from build123d import *

# Parameters (mm, degrees)
SKETCH1_W           = 25.27
SKETCH1_H           = 23.36
SKETCH1_R           = 1.5
SKETCH1_W_2         = 12.27
SKETCH1_H_2         = 10.36
SKETCH1_W_3         = 4
BOSS_EXTRUDE1_DEPTH = 3


with BuildPart() as part:
    # Sketch1 → Boss-Extrude1 (new body)
    # profile 1 of 2: a face of its own
    with BuildSketch(Plane.XY):
        Rectangle(SKETCH1_W, SKETCH1_H)
        with Locations((-9.635, 8.68)):
            Circle(SKETCH1_R, mode=Mode.SUBTRACT)
        with Locations((-9.635, -8.68)):
            Circle(SKETCH1_R, mode=Mode.SUBTRACT)
        with Locations((9.635, -8.68)):
            Circle(SKETCH1_R, mode=Mode.SUBTRACT)
        with Locations((9.635, 8.68)):
            Circle(SKETCH1_R, mode=Mode.SUBTRACT)
        with Locations((-0.085, -0.04)):
            Rectangle(SKETCH1_W_2, SKETCH1_H_2, mode=Mode.SUBTRACT)
    # profile 2 of 2: a face of its own
    with BuildSketch(Plane.XY):
        with Locations((-0.635, -0.04)):
            Rectangle(SKETCH1_W_3, SKETCH1_H_2)
    extrude(amount=BOSS_EXTRUDE1_DEPTH)


solid = part.part
The listing builds one solid part. Answer for the finished solid, in the listing's coordinates (mm). A direction names the side the tool comes from. Round coordinates to 2 decimals unless told otherwise and drop trailing zeros. Write each loop counter-clockwise with the first axis right and the second up, starting at its lowest first coordinate (ties: lowest second). Pieces come first, ordered by that corner, then holes. Notation, with made-up numbers: M 69,-33 L 124,-33 A16 cw 124,-7 Z; hole C 68.5,73.25 d2. An arc over 180 degrees is marked long. Write each question's results on one line, items separated by ' | '. Start each with the question number.
Item 1: A cutting plane is placed at A-A on y = 2.5. Write down the section's boundary in (x, z) (3 decimals).
Item 2: A cutting plane is placed at B-B on x = 3.5. Write down the section's boundary in (y, z), and give its area (3 significant figures).
Item 3: For a pull along X with two mould halves and no side action, classify faces 1 (the face through (12.635, 0, 1)), 2 (the face through (0, 0, 0)), 3 (the face through (-9.96, -10.144, 1.479)) as pulls with the +X half, pulls with the -X half, needs draft (parallel to the pull), parting line crosses it, or undercut.
Item 4: A cutting plane is placed at C-C on z = 0.95. Write down the section's boundary in (x, y) (3 decimals).
Item 5: Straight lines are drawn through the part: L1, parallel to X at y = 0.5, z = 1 (3 decimals); L2, parallel to Y at x = 9.75, z = 1.6; L3, parallel to Y at x = 5, z = 2.05. For each, find the intervals that lie inside material, in ascending order. Write a range as [from, to].
Item 6: A flat-ended cylindrical pin translates along its axis: pin 1 Ø1.8 at (x, y) = (9.635, -8.68) entering from -Z. Find the tip coordinate at first contact, or state that the pin passes through.
Item 7: For faces 4 (the face through (0, 0, 3)), 5 (the face through (-4, -5.22, 1)), determine the directions among +Z, -Z, +X, -X, +Y, -Y from which every point of the face is accessible in a straight line to the end or side of a thin tool.
Item 8: A cutting plane is placed at D-D on y = -8.68. Write down the section's boundary in (x, z) (3 decimals), and give its area (3 significant figures).
Check sheet entries:
1) outline: M -12.635,0 L -6.22,0 L -6.22,3 L -12.635,3 Z; M -2.635,0 L 1.365,0 L 1.365,3 L -2.635,3 Z; M 6.05,0 L 12.635,0 L 12.635,3 L 6.05,3 Z
2) outline: M -11.68,0 L -5.22,0 L -5.22,3 L -11.68,3 Z; M 5.14,0 L 11.68,0 L 11.68,3 L 5.14,3 Z | area: 39.0 mm²
3) face 1: pulls with the +X half | face 2: needs draft | face 3: undercut
4) outline: M -12.635,-11.68 L 12.635,-11.68 L 12.635,11.68 L -12.635,11.68 Z; hole C -9.635,-8.68 d3; hole C -9.635,8.68 d3; hole M -6.22,-5.22 L -2.635,-5.22 L -2.635,5.14 L -6.22,5.14 Z; hole M 1.365,-5.22 L 6.05,-5.22 L 6.05,5.14 L 1.365,5.14 Z; hole C 9.635,-8.68 d3; hole C 9.635,8.68 d3
5) L1: [-12.635, -6.22], [-2.635, 1.365], [6.05, 12.635] | L2: [-11.68, -10.18], [-7.18, 7.18], [10.18, 11.68] | L3: [-11.68, -5.22], [5.14, 11.68]
6) pin 1: through
7) face 4: +Z, +X, -X, +Y, -Y | face 5: +Z, -Z
8) outline: M -12.635,0 L -11.135,0 L -11.135,3 L -12.635,3 Z; M -8.135,0 L 8.135,0 L 8.135,3 L -8.135,3 Z; M 11.135,0 L 12.635,0 L 12.635,3 L 11.135,3 Z | area: 57.8 mm²
